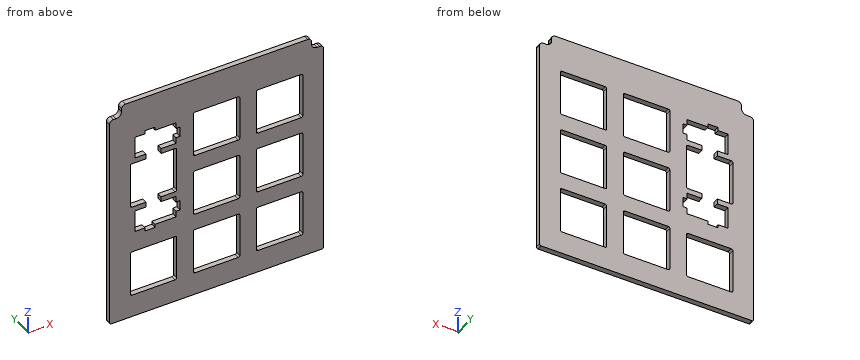
from build123d import *

# Parameters (mm, degrees)
EXTRUDE_1_DEPTH                = 1.6
SKETCH_2_W                     = 14
SKETCH_2_H                     = 14
CUT_EXTRUDE_1_DEPTH            = 1.6
FILLET_1_R                     = 0.5
PATTERN_LINEAR_2_COUNT         = 3
PATTERN_LINEAR_2_PITCH         = 19
PATTERN_LINEAR_2_COUNT_DIR2    = 3
PATTERN_LINEAR_2_PITCH_DIR2    = 19
FILLET_1_OF_PATTERN_LINEAR_2_R = 0.5
CUT_EXTRUDE_3_DEPTH            = 1.6
FILLET_2_R                     = 0.5


with BuildPart() as part:
    # 草图1 → 凸台-拉伸1 (new body)
    with BuildSketch(Plane(origin=(0, 0, 0), x_dir=(1, 0, 0), z_dir=(0, 1, 0))):
        with BuildLine():
            Line((-12.500806884, 61.22832279), (51.999193116, 61.22832279))
            Line((51.999193116, 61.22832279), (51.999193116, -3.47167721))
            ThreePointArc((51.999193116, -3.47167721), (51.662365914, -4.284850009), (50.849193116, -4.62167721))
            Line((50.849193116, -4.62167721), (49.999193116, -4.62167721))
            ThreePointArc((49.999193116, -4.62167721), (48.832466927, -5.104951021), (48.349193116, -6.27167721))
            Line((48.349193116, -6.27167721), (48.349193116, -7.12167721))
            ThreePointArc((48.349193116, -7.12167721), (48.012365914, -7.934850009), (47.199193116, -8.27167721))
            Line((47.199193116, -8.27167721), (-7.700806884, -8.27167721))
            ThreePointArc((-7.700806884, -8.27167721), (-8.513979683, -7.934850009), (-8.850806884, -7.12167721))
            Line((-8.850806884, -7.12167721), (-8.850806884, -6.27167721))
            ThreePointArc((-8.850806884, -6.27167721), (-9.334080695, -5.104951021), (-10.500806884, -4.62167721))
            Line((-10.500806884, -4.62167721), (-11.350806884, -4.62167721))
            ThreePointArc((-11.350806884, -4.62167721), (-12.163979683, -4.284850009), (-12.500806884, -3.47167721))
            Line((-12.500806884, -3.47167721), (-12.500806884, 61.22832279))
        make_face()
    extrude(amount=EXTRUDE_1_DEPTH)

    # 草图2 → 切除-拉伸1 (cut)
    with BuildSketch(Plane.XZ):
        with Locations((38.749193116, -9.315811453)):
            Rectangle(SKETCH_2_W, SKETCH_2_H)
    cut_extrude_1 = extrude(amount=-CUT_EXTRUDE_1_DEPTH, mode=Mode.SUBTRACT)

    # 圆角1
    fillet_1_edges = [part.edges().sort_by_distance(p)[0] for p in [
        (31.749193116, 0.8, -16.315811453),
        (31.749193116, 0.8, -2.315811453),
        (45.749193116, 0.8, -2.315811453),
        (45.749193116, 0.8, -16.315811453),
    ]]
    fillet(fillet_1_edges, radius=FILLET_1_R)

    # 阵列(线性)2: Cut-Extrude 1 3 × 3, 2 skipped
    with Locations(*[(-j * PATTERN_LINEAR_2_PITCH_DIR2, 0, -i * PATTERN_LINEAR_2_PITCH) for i in range(PATTERN_LINEAR_2_COUNT) for j in range(PATTERN_LINEAR_2_COUNT_DIR2) if (i, j) not in ((0, 0), (0, 2), (1, 2))]):
        add(cut_extrude_1, mode=Mode.SUBTRACT)

    # 圆角1 of 阵列(线性)2
    fillet_1_of_pattern_linear_2_edges = [part.edges().sort_by_distance(p)[0] for p in [
        (12.749193116, 0.8, -16.315811453),
        (12.749193116, 0.8, -2.315811453),
        (26.749193116, 0.8, -2.315811453),
        (26.749193116, 0.8, -16.315811453),
        (31.749193116, 0.8, -35.315811453),
        (31.749193116, 0.8, -21.315811453),
        (45.749193116, 0.8, -21.315811453),
        (45.749193116, 0.8, -35.315811453),
        (12.749193116, 0.8, -35.315811453),
        (12.749193116, 0.8, -21.315811453),
        (26.749193116, 0.8, -21.315811453),
        (26.749193116, 0.8, -35.315811453),
        (31.749193116, 0.8, -54.315811453),
        (31.749193116, 0.8, -40.315811453),
        (45.749193116, 0.8, -40.315811453),
        (45.749193116, 0.8, -54.315811453),
        (12.749193116, 0.8, -54.315811453),
        (12.749193116, 0.8, -40.315811453),
        (26.749193116, 0.8, -40.315811453),
        (26.749193116, 0.8, -54.315811453),
        (-6.250806884, 0.8, -54.315811453),
        (-6.250806884, 0.8, -40.315811453),
        (7.749193116, 0.8, -40.315811453),
        (7.749193116, 0.8, -54.315811453),
    ]]
    fillet(fillet_1_of_pattern_linear_2_edges, radius=FILLET_1_OF_PATTERN_LINEAR_2_R)

    # 草图3 → 切除-拉伸3 (cut)
    with BuildSketch(Plane(origin=(0, 1.6, 0), x_dir=(1, 0, 0), z_dir=(0, 1, 0))):
        with BuildLine():
            Line((-6.250806884, 12.315811453), (-6.250806884, 25.315811453))
            ThreePointArc((-6.250806884, 25.315811453), (-6.104360275, 25.669364844), (-5.750806884, 25.815811453))
            Line((-5.750806884, 25.815811453), (-1.550806884, 25.815811453))
            Line((-1.550806884, 25.815811453), (-1.550806884, 27.395811453))
            Line((-1.550806884, 27.395811453), (-4.780806884, 27.395811453))
            Line((-4.780806884, 27.395811453), (-4.780806884, 34.045811453))
            Line((-4.780806884, 34.045811453), (-1.750806884, 34.045811453))
            Line((-1.750806884, 34.045811453), (-1.750806884, 35.045811453))
            Line((-1.750806884, 35.045811453), (1.249193116, 35.045811453))
            Line((1.249193116, 35.045811453), (1.249193116, 34.045811453))
            Line((1.249193116, 34.045811453), (7.519193116, 34.045811453))
            Line((7.519193116, 34.045811453), (7.519193116, 32.220811453))
            Line((7.519193116, 32.220811453), (8.719193116, 32.220811453))
            Line((8.719193116, 32.220811453), (8.719193116, 29.220811453))
            Line((8.719193116, 29.220811453), (7.519193116, 29.220811453))
            Line((7.519193116, 29.220811453), (7.519193116, 27.395811453))
            Line((7.519193116, 27.395811453), (3.049193116, 27.395811453))
            Line((3.049193116, 27.395811453), (3.049193116, 25.815811453))
            Line((3.049193116, 25.815811453), (7.249193116, 25.815811453))
            ThreePointArc((7.249193116, 25.815811453), (7.602746506, 25.669364844), (7.749193116, 25.315811453))
            Line((7.749193116, 25.315811453), (7.749193116, 12.315811453))
            ThreePointArc((7.749193116, 12.315811453), (7.602746506, 11.962258063), (7.249193116, 11.815811453))
            Line((7.249193116, 11.815811453), (3.049193116, 11.815811453))
            Line((3.049193116, 11.815811453), (3.049193116, 10.235811453))
            Line((3.049193116, 10.235811453), (7.519193116, 10.235811453))
            Line((7.519193116, 10.235811453), (7.519193116, 8.410811453))
            Line((7.519193116, 8.410811453), (8.719193116, 8.410811453))
            Line((8.719193116, 8.410811453), (8.719193116, 5.410811453))
            Line((8.719193116, 5.410811453), (7.519193116, 5.410811453))
            Line((7.519193116, 5.410811453), (7.519193116, 3.585811453))
            Line((7.519193116, 3.585811453), (1.249193116, 3.585811453))
            Line((1.249193116, 3.585811453), (1.249193116, 2.585811453))
            Line((1.249193116, 2.585811453), (-1.750806884, 2.585811453))
            Line((-1.750806884, 2.585811453), (-1.750806884, 3.585811453))
            Line((-1.750806884, 3.585811453), (-4.780806884, 3.585811453))
            Line((-4.780806884, 3.585811453), (-4.780806884, 10.235811453))
            Line((-4.780806884, 10.235811453), (-1.550806884, 10.235811453))
            Line((-1.550806884, 10.235811453), (-1.550806884, 11.815811453))
            Line((-1.550806884, 11.815811453), (-5.750806884, 11.815811453))
            ThreePointArc((-5.750806884, 11.815811453), (-6.104360275, 11.962258063), (-6.250806884, 12.315811453))
        make_face()
    extrude(amount=-CUT_EXTRUDE_3_DEPTH, mode=Mode.SUBTRACT)

    # 圆角2
    fillet_2_edges = [part.edges().sort_by_distance(p)[0] for p in [
        (-12.500806884, 0.8, -61.22832279),
        (51.999193116, 0.8, -61.22832279),
    ]]
    fillet(fillet_2_edges, radius=FILLET_2_R)


solid = part.part
Input: part model. Units: mm. Frame: model coordinates. Coordinates: 2 decimals unless noted, no trailing zeros. Loops run counter-clockwise (first coordinate to the right, second up) from the corner with the lowest first, then second, coordinate; pieces in that order, holes last. Notation, with made-up numbers: (-30, -31.5) - (21, -31.5) arc R20 ccw to (21, -2.5) - close; hole circle Ø5 at (-30.5, -22). An arc over 180 degrees is marked (long way). Answer in a Markdown table with one row per item. Add a question column.
Item 1: Section query A-A on x = 44. Return the cut outline in (y, z), then the cut area to 3 significant figures.
Item 2: Line query: line 1 along X through (y, z) = (0.45, -4); line 2 along Z through (x, y) = (40, 1.25); line 3 along X through (y, z) = (1.4, -8). Output: solid intervals per line, ascending. Write a range as [from, to].
Item 3: Contact query for a flat-ended pin moving along its axis: P1, Ø8, axis at x = 6.5, z = -3.5, coming from the -Y side. Output: stop coordinate, or through.
Item 4: Section query C-C on y = 0.85. State how many separate pieces and enclosed holes the cut face has, then the cut area to 3 significant figures.
Item 5: Section query B-B on z = -47. Return the cut outline in (x, y), then the cut area to 3 significant figures.
Recorded:
| question | item | result |
|---|---|---|
| 1 | outline | (0, -61.23) - (1.6, -61.23) - (1.6, -54.32) - (0, -54.32) - close; (0, -40.32) - (1.6, -40.32) - (1.6, -35.32) - (0, -35.32) - close; (0, -21.32) - (1.6, -21.32) - (1.6, -16.32) - (0, -16.32) - close; (0, -2.32) - (1.6, -2.32) - (1.6, 8.27) - (0, 8.27) - close |
| 1 | area | 44.0 mm^2 |
| 2 | line 1 | [-12.5, -4.78], [7.52, 12.75], [26.75, 31.75], [45.75, 52] |
| 2 | line 2 | [-61.23, -54.32], [-40.32, -35.32], [-21.32, -16.32], [-2.32, 8.27] |
| 2 | line 3 | [-12.5, -4.78], [8.72, 12.75], [26.75, 31.75], [45.75, 52] |
| 3 | P1 | y = 0 |
| 4 | separate pieces | 1 |
| 4 | enclosed holes | 8 |
| 4 | area | 2,700 mm^2 |
| 5 | outline | (-12.5, 0) - (-6.25, 0) - (-6.25, 1.6) - (-12.5, 1.6) - close; (7.75, 0) - (12.75, 0) - (12.75, 1.6) - (7.75, 1.6) - close; (26.75, 0) - (31.75, 0) - (31.75, 1.6) - (26.75, 1.6) - close; (45.75, 0) - (52, 0) - (52, 1.6) - (45.75, 1.6) - close |
| 5 | area | 36.0 mm^2 |
